from build123d import *

# Parameters (mm, degrees)
SKETCH_1_W          = 58
SKETCH_1_H          = 70
EXTRUDE_1_DEPTH     = 18.9
CUT_EXTRUDE_1_DEPTH = 17
SKETCH_2_3_R        = 1.7
CUT_EXTRUDE_2_DEPTH = 4
FILLET_1_R          = 1
FILLET_2_R          = 2
SKETCH_4_R          = 1.5
CUT_EXTRUDE_3_DEPTH = 2
SKETCH_4_3_W        = 15
SKETCH_4_3_H        = 4
SKETCH_4_3_W_2      = 4
SKETCH_4_3_H_2      = 6
SKETCH_4_3_W_3      = 9
EXTRUDE_2_DEPTH     = 10
SKETCH_7_R          = 5.4
CUT_EXTRUDE_4_DEPTH = 2
CUT_EXTRUDE_5_DEPTH = 2
EXTRUDE_3_DEPTH     = 1.5


with BuildPart() as part:
    # Sketch 1 → Extrude 1 (new body)
    with BuildSketch(Plane.XY):
        Rectangle(SKETCH_1_W, SKETCH_1_H)
    extrude(amount=EXTRUDE_1_DEPTH)

    # Sketch 2 → Cut-Extrude 1 (cut)
    with BuildSketch(Plane.XY.offset(18.9)):
        Polygon((-27, 29), (-27, -33), (23, -33), (23, -29), (27, -29), (27, 29), (23, 29), (23, 33), (-23, 33), (-23, 29), align=None)
    extrude(amount=-CUT_EXTRUDE_1_DEPTH, mode=Mode.SUBTRACT)

    # Sketch 2_3 → Cut-Extrude 2 (cut)
    with BuildSketch(Plane.XY.offset(18.9)):
        with Locations((-26, 32)):
            Circle(SKETCH_2_3_R)
        with Locations(Location((26, 32, 0), (0, 0, 180))):
            Circle(SKETCH_2_3_R)
        with Locations((26, -32)):
            Circle(SKETCH_2_3_R)
        with Locations((-26, -32)):
            Circle(SKETCH_2_3_R)
    extrude(amount=-CUT_EXTRUDE_2_DEPTH, mode=Mode.SUBTRACT)

    # Fillet 1
    fillet_1_edges = [part.edges().sort_by_distance(p)[0] for p in [
        (-27, 29, 10.4),
        (-23, 29, 10.4),
        (-23, 33, 10.4),
        (23, 33, 10.4),
        (23, 29, 10.4),
        (27, 29, 10.4),
        (27, -29, 10.4),
        (23, -29, 10.4),
        (23, -33, 10.4),
    ]]
    fillet(fillet_1_edges, radius=FILLET_1_R)

    # Fillet 2
    fillet_2_edges = [part.edges().sort_by_distance(p)[0] for p in [
        (0, -35, 0),
        (-29, 0, 0),
        (0, 35, 0),
        (29, 0, 0),
        (29, -35, 9.45),
        (-29, -35, 9.45),
        (-29, 35, 9.45),
        (29, 35, 9.45),
    ]]
    fillet(fillet_2_edges, radius=FILLET_2_R)

    # Sketch 4 → Cut-Extrude 3 (cut)
    with BuildSketch(Plane.XY.offset(1.9)):
        with Locations((-20.9, 21.7)):
            Circle(SKETCH_4_R)
    extrude(amount=-CUT_EXTRUDE_3_DEPTH, mode=Mode.SUBTRACT)

    # Sketch 4_3 → Extrude 2 (add)
    with BuildSketch(Plane.XY.offset(1.9)):
        with Locations((5.5, -31)):
            Rectangle(SKETCH_4_3_W, SKETCH_4_3_H)
        with Locations((-25, 10)):
            Rectangle(SKETCH_4_3_W_2, SKETCH_4_3_H_2)
        with Locations((9.5, 30)):
            Rectangle(SKETCH_4_3_W_3, SKETCH_4_3_H_2)
    extrude(amount=EXTRUDE_2_DEPTH)

    # Sketch 7 → Cut-Extrude 4 (cut)
    with BuildSketch(Plane.ZY.offset(29)):
        with Locations(Location((7.3, 0, 0), (0, 0, 191.043665527))):
            Circle(SKETCH_7_R)
    extrude(amount=-CUT_EXTRUDE_4_DEPTH, mode=Mode.SUBTRACT)

    # Sketch 8 → Cut-Extrude 5 (cut)
    with BuildSketch(Plane.XZ.offset(35)):
        with BuildLine():
            Line((-21.65, 6.65), (-15.95, 6.65))
            ThreePointArc((-15.95, 6.65), (-14.3, 5), (-15.95, 3.35))
            Line((-15.95, 3.35), (-21.65, 3.35))
            ThreePointArc((-21.65, 3.35), (-23.3, 5), (-21.65, 6.65))
        make_face()
    extrude(amount=-CUT_EXTRUDE_5_DEPTH, mode=Mode.SUBTRACT)

    # Sketch 10 → Extrude 3 (add)
    with BuildSketch(Plane.XY.offset(1.9)):
        Polygon((-9.3, -7.1), (-9.3, -33), (-7.8, -33), (-7.8, -5.6), (-27, -5.6), (-27, -7.1), align=None)
    extrude(amount=EXTRUDE_3_DEPTH)


solid = part.part
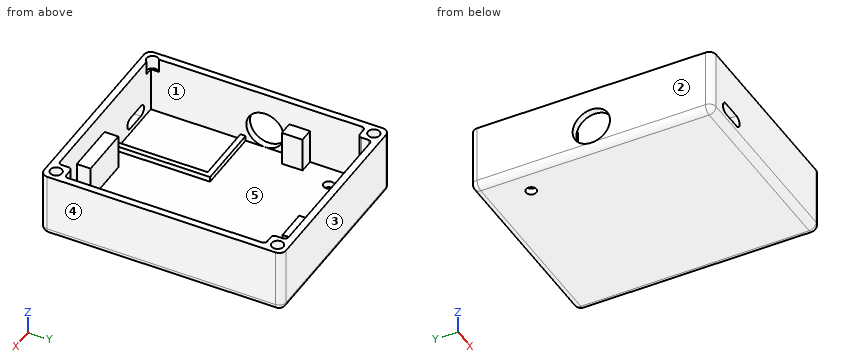
Verification items for the finished model (mm, model axes). Face numbers are marked on the shaded views. A direction names the side the tool comes from. Coordinates: 2 decimals unless noted, no trailing zeros. Order: outer loops, then holes, each group sorted by start corner. A loop starts at its lowest first (then second) coordinate and runs counter-clockwise, first axis right, second up. Notation, with made-up numbers: M 15,-17 L 40,-17 A28 ccw 40,18 Z; hole C -38.75,11 d1. An arc over 180 degrees is marked long. Return JSON: item names as keys, results as strings.
1) Cross-section at A-A, the plane y = 21.7. Record the boundary of the cut face in (x, z), and give its area (3 significant figures).
Answer list:
{"outline": "M -29,2 A2 ccw -27,0 L -22.4,0 L -22.4,1.9 L -27,1.9 L -27,18.9 L -29,18.9 Z; M -19.4,0 L 27,0 A2 ccw 29,2 L 29,18.9 L 27,18.9 L 27,1.9 L -19.4,1.9 Z", "area": "171 mm2"}
2) Cross-section at C-C, the plane y = 8.5. Record the boundary of the cut face in (x, z).
Answer list:
{"outline": "M -29,2 A2 ccw -27,0 L 27,0 A2 ccw 29,2 L 29,18.9 L 27,18.9 L 27,1.9 L -23,1.9 L -23,11.9 L -27,11.9 L -27,18.9 L -29,18.9 Z"}
3) Access from +Z, -Z, +X, -X, +Y, -Y to the whole of each face (thin tool, end or side, straight path). Record for the marked faces 1 and 2.
Answer list:
{"face 1": "+Z", "face 2": "+Z, -Z, -X, +Y, -Y"}
4) Release check for a two-part mould opening along Y. For the marked faces 3, 4 and 5 record: +Y half, -Y half, draft (parallel to the pull), parting line (faces both ways), or undercut.
Answer list:
{"face 3": "+Y half", "face 4": "draft", "face 5": "undercut"}
5) Cross-section at B-B, the plane x = 3. Record the boundary of the cut face in (y, z).
Answer list:
{"outline": "M -35,2 A2 ccw -33,0 L 33,0 A2 ccw 35,2 L 35,18.9 L 33,18.9 L 33,1.9 L -29,1.9 L -29,11.9 L -33,11.9 L -33,18.9 L -35,18.9 Z"}
6) Cross-section at D-D, the plane x = 20.5. Record the boundary of the cut face in (y, z).
Answer list:
{"outline": "M -35,2 A2 ccw -33,0 L 33,0 A2 ccw 35,2 L 35,18.9 L 33,18.9 L 33,1.9 L -33,1.9 L -33,18.9 L -35,18.9 Z"}
7) Thickness scan on L1, parallel to Y at x = -26, z = 16.8; L2, parallel to X at y = 31, z = 3.25; L3, parallel to Y at x = 26, z = 17.9. Record the ranges inside material, lowest first. Write a range as [from, to].
Answer list:
{"L1": "[-35, -33.7], [29, 30.3], [33.7, 35]", "L2": "[-29, -23], [5, 14], [23, 29]", "L3": "[-35, -33.7], [-30.3, -29], [29, 30.3], [33.7, 35]"}
8) Gauge pin test, flat ends, axial feed: pin 1 (12 mm diameter, centred on x = 4, y = -15, fed in from +Z); pin 2 (2.5 mm diameter, centred on x = -26, y = 32, fed in from +Z); pin 3 (5.5 mm diameter, centred on x = 26, y = 32, fed in from +Z). Record the tip position at first contact, or that the pin passes through.
Answer list:
{"pin 1": "z = 1.9", "pin 2": "z = 14.9", "pin 3": "z = 18.9"}
